Source: three-view drawing plus pictorial views. Frame: mm from the lowest corner of the part. A direction names the side the tool comes from. Give positions to 0.01 mm unless a question says otherwise; leave off trailing zeros. Loops run counter-clockwise (first coordinate to the right, second up) from the corner with the lowest first, then second, coordinate; pieces in that order, holes last. Notation, with made-up numbers: (26.5, -37) - (73.5, -37) arc R22 cw to (73.5, -8) - close; hole circle Ø8 at (81.25, 24). An arc over 180 degrees is marked (long way). Answer as a JSON object with one key per item and string values.
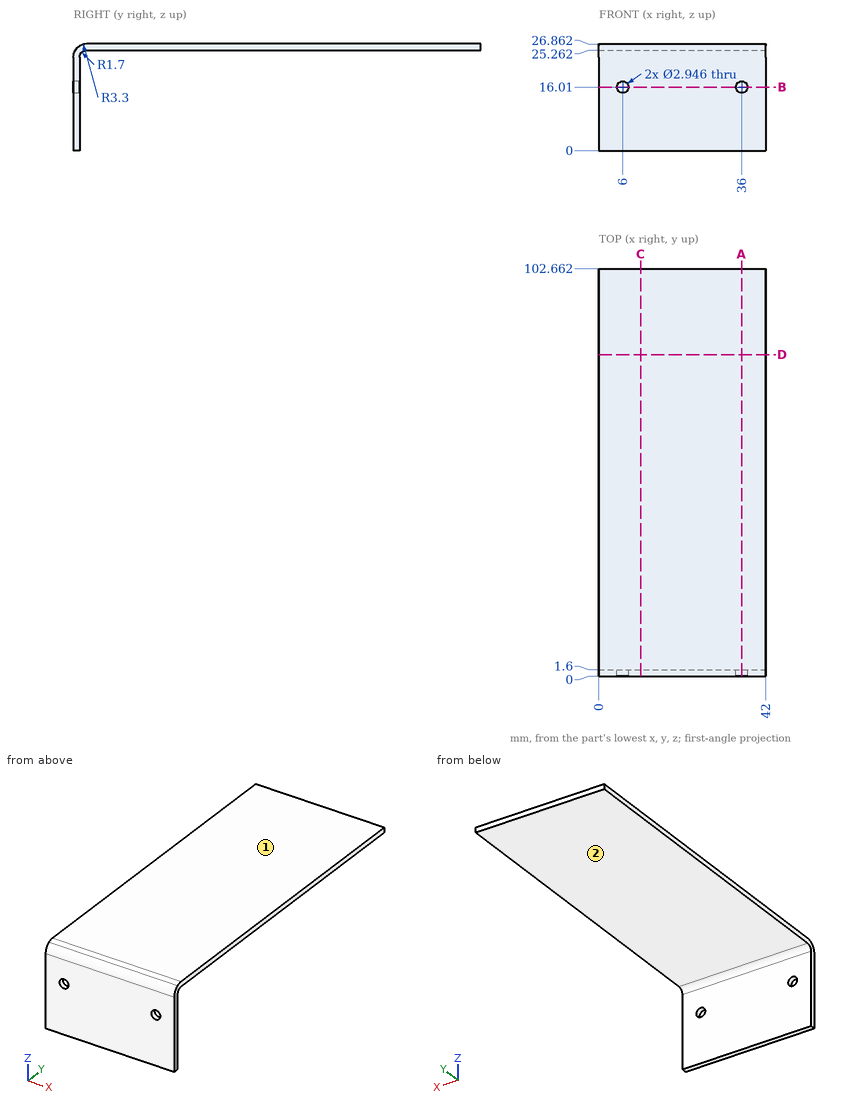
Item 1: Access query for the marked faces 1 and 2. Directions: +Z, -Z, +X, -X, +Y, -Y. A direction counts if a zero-diameter tool reaches every point of the face in a straight line with its end or side. Return the directions, or none.
Geometry check:
{"face 1": "+Z, +X, -X, +Y, -Y", "face 2": "-Z, +X, -X, +Y"}
Item 2: Cut plane A-A (x = 36). Return loops of the section in (y, z).
Geometry check:
{"outline": "(0, 0) - (1.6, 0) - (1.6, 14.54) - (0, 14.54) - close; (0, 17.48) - (1.6, 17.48) - (1.6, 23.56) arc R1.7 cw to (3.3, 25.26) - (102.66, 25.26) - (102.66, 26.86) - (3.3, 26.86) arc R3.3 ccw to (0, 23.56) - close"}
Item 3: Contact query for flat-ended pins moving along their axis: P1, Ø5, axis at x = 22.5, z = 14.5, coming from the +Y side; P2, Ø2, axis at x = 13, y = 20.5, coming from the -Z side. Output: stop coordinate, or through.
Geometry check:
{"P1": "stops at y = 1.6", "P2": "stops at z = 25.26"}
Item 4: Cut plane D-D (y = 81). Return loops of the section in (x, z).
Geometry check:
{"outline": "(0, 25.26) - (42, 25.26) - (42, 26.86) - (0, 26.86) - close"}
Item 5: Cut plane C-C (x = 10.5). Return loops of the section in (y, z).
Geometry check:
{"outline": "(0, 0) - (1.6, 0) - (1.6, 23.56) arc R1.7 cw to (3.3, 25.26) - (102.66, 25.26) - (102.66, 26.86) - (3.3, 26.86) arc R3.3 ccw to (0, 23.56) - close"}
Item 6: Cut plane B-B (z = 16.01). Return loops of the section in (x, y).
Geometry check:
{"outline": "(0, 0) - (4.53, 0) - (4.53, 1.6) - (0, 1.6) - close; (7.47, 0) - (34.53, 0) - (34.53, 1.6) - (7.47, 1.6) - close; (37.47, 0) - (42, 0) - (42, 1.6) - (37.47, 1.6) - close"}
Item 7: Material intervals for line 1 (X direction, y = 0.7, z = 16.01); line 2 (Y direction, x = 38, z = 21.25); line 3 (Z direction, x = 13, y = 95.5), sorted ascending. Write a range as [from, to].
Geometry check:
{"line 1": "x = [0, 4.53], [7.47, 34.53], [37.47, 42]", "line 2": "y = [0, 1.6]", "line 3": "z = [25.26, 26.86]"}
